```python
from build123d import *

# Parameters (mm, degrees)
SKETCH1_W           = 60
SKETCH1_H           = 60
SKETCH1_R           = 2.95
SKETCH1_R_2         = 2.25
BOSS_EXTRUDE1_DEPTH = 6.35
FILLET1_R           = 5


with BuildPart() as part:
    # Sketch1 → Boss-Extrude1 (new body)
    with BuildSketch(Plane(origin=(0, 0, 0), x_dir=(1, 0, 0), z_dir=(0, 1, 0))):
        with Locations((30, 30)):
            Rectangle(SKETCH1_W, SKETCH1_H)
        with Locations(Location((14, 48, 0), (0, 0, 270))):
            Circle(SKETCH1_R, mode=Mode.SUBTRACT)
        with Locations(Location((46, 48, 0), (0, 0, 270))):
            Circle(SKETCH1_R, mode=Mode.SUBTRACT)
        with Locations(Location((46, 12, 0), (0, 0, 270))):
            Circle(SKETCH1_R, mode=Mode.SUBTRACT)
        with Locations(Location((14, 12, 0), (0, 0, 270))):
            Circle(SKETCH1_R, mode=Mode.SUBTRACT)
        with Locations(Location((56, 8, 0), (0, 0, 270))):
            Circle(SKETCH1_R_2, mode=Mode.SUBTRACT)
        with Locations(Location((4, 8, 0), (0, 0, 90))):
            Circle(SKETCH1_R_2, mode=Mode.SUBTRACT)
        with Locations(Location((55, 16, 0), (0, 0, 270))):
            Circle(SKETCH1_R_2, mode=Mode.SUBTRACT)
        with Locations(Location((55, 24, 0), (0, 0, 270))):
            Circle(SKETCH1_R_2, mode=Mode.SUBTRACT)
        with Locations(Location((55, 32, 0), (0, 0, 270))):
            Circle(SKETCH1_R_2, mode=Mode.SUBTRACT)
        with Locations(Location((5, 32, 0), (0, 0, 90))):
            Circle(SKETCH1_R_2, mode=Mode.SUBTRACT)
        with Locations(Location((5, 24, 0), (0, 0, 90))):
            Circle(SKETCH1_R_2, mode=Mode.SUBTRACT)
        with Locations(Location((5, 16, 0), (0, 0, 90))):
            Circle(SKETCH1_R_2, mode=Mode.SUBTRACT)
    extrude(amount=BOSS_EXTRUDE1_DEPTH)

    # Fillet1
    fillet1_edges = [part.edges().sort_by_distance(p)[0] for p in [
        (0, 3.175, -60),
        (60, 3.175, -60),
        (60, 3.175, 0),
        (0, 3.175, 0),
    ]]
    fillet(fillet1_edges, radius=FILLET1_R)


solid = part.part
```
Could you check a few things on this model? Use its own coordinates, in mm. Coordinates: 2 decimals unless noted, no trailing zeros. Write each loop counter-clockwise with the first axis right and the second up, starting at its lowest first coordinate (ties: lowest second). Pieces come first, ordered by that corner, then holes. Notation, with made-up numbers: (64, 51.5) -> (118, 51.5) arc R17 ccw to (118, 65.5) -> close; hole circle Ø5 at (30, 31.5). An arc over 180 degrees is marked (long way). Return JSON: item names as keys, results as strings.
(1) Imagine slicing it at C-C, the plane y = 4.75. Count the separate pieces of the cut face and the enclosed holes in it, then the cut area to 3 significant figures.
Numbers:
{"separate pieces": "1", "enclosed holes": "12", "area": "3,340 mm2"}
(2) Imagine slicing it at B-B, the plane x = 14. Please give me the cut outline in (y, z).
Numbers:
{"outline": "(0, -60) -> (6.35, -60) -> (6.35, -50.95) -> (0, -50.95) -> close; (0, -45.05) -> (6.35, -45.05) -> (6.35, -14.95) -> (0, -14.95) -> close; (0, -9.05) -> (6.35, -9.05) -> (6.35, 0) -> (0, 0) -> close"}
(3) I need wall thicknesses on L1, parallel to X at y = 1.5, z = -32; L2, parallel to Z at x = 15, y = 1; L3, parallel to Z at x = 4.5, y = 4. Which ranges of each line are inside material? Lowest first, please.
Numbers:
{"L1": "x = 0 to 2.75, 7.25 to 52.75, 57.25 to 60", "L2": "z = -60 to -50.78, -45.22 to -14.78, -9.22 to 0", "L3": "z = -59.97 to -34.19, -29.81 to -26.19, -21.81 to -18.19, -13.81 to -10.19, -5.81 to -0.03"}
(4) Imagine slicing it at A-A, the plane z = -16. Please give me the cut outline in (x, y).
Numbers:
{"outline": "(0, 0) -> (2.75, 0) -> (2.75, 6.35) -> (0, 6.35) -> close; (7.25, 0) -> (52.75, 0) -> (52.75, 6.35) -> (7.25, 6.35) -> close; (57.25, 0) -> (60, 0) -> (60, 6.35) -> (57.25, 6.35) -> close"}
(5) We'd pull the mould along X, two halves only. Please class faces 1 (the cylindrical face through (1, 3, -58)), 2 (the cylindrical face through (56.897, 3.131, -22.79)), 3 (the flat face through (30, 3, -60)): +X half, -X half, draft (parallel to the pull), parting line (faces both ways), or undercut.
Numbers:
{"face 1": "-X half", "face 2": "undercut", "face 3": "draft"}
(6) Imagine slicing it at D-D, the plane x = 56. Please give me the cut outline in (y, z), then the cut area to 3 significant figures.
Numbers:
{"outline": "(0, -59.9) -> (6.35, -59.9) -> (6.35, -34.02) -> (0, -34.02) -> close; (0, -29.98) -> (6.35, -29.98) -> (6.35, -26.02) -> (0, -26.02) -> close; (0, -21.98) -> (6.35, -21.98) -> (6.35, -18.02) -> (0, -18.02) -> close; (0, -13.98) -> (6.35, -13.98) -> (6.35, -10.25) -> (0, -10.25) -> close; (0, -5.75) -> (6.35, -5.75) -> (6.35, -0.1) -> (0, -0.1) -> close", "area": "274 mm2"}
